```python
from build123d import *

# Parameters (mm, degrees)
SKETCH1_W            = 300
SKETCH1_H            = 20
BOSS_EXTRUDE1_DEPTH  = 8
SKETCH2_W            = 34
SKETCH2_H            = 8
BOSS_EXTRUDE2_DEPTH  = 9
SKETCH3_W            = 34
SKETCH3_H            = 8
BOSS_EXTRUDE3_DEPTH  = 9
SKETCH4_R            = 1.65
CUT_EXTRUDE1_DEPTH   = 302.504560496
SKETCH5_W            = 25
SKETCH5_H            = 8
BOSS_EXTRUDE4_DEPTH  = 17
SKETCH6_W            = 25
SKETCH6_H            = 8
BOSS_EXTRUDE5_DEPTH  = 17
SKETCH7_W            = 10
SKETCH7_H            = 38
CUT_EXTRUDE2_DEPTH   = 303.37890138
SKETCH8_W            = 7
SKETCH8_H            = 16
CUT_EXTRUDE3_DEPTH   = 4
CUT_EXTRUDE4_DEPTH   = 7
BOSS_EXTRUDE6_DEPTH  = 10
SKETCH12_W           = 8
SKETCH12_H           = 8
BOSS_EXTRUDE7_DEPTH  = 17
SKETCH13_R           = 1.7
CUT_EXTRUDE6_DEPTH   = 305.926220585
SKETCH14_W           = 20
SKETCH14_H           = 13
BOSS_EXTRUDE8_DEPTH  = 12
SKETCH15_R           = 1.6
CUT_EXTRUDE7_DEPTH   = 20
SKETCH16_W           = 20
SKETCH16_H           = 13
BOSS_EXTRUDE9_DEPTH  = 12
SKETCH17_R           = 1.6
CUT_EXTRUDE8_DEPTH   = 20
SKETCH18_W           = 20
SKETCH18_H           = 13
BOSS_EXTRUDE10_DEPTH = 12
SKETCH19_R           = 1.65
CUT_EXTRUDE9_DEPTH   = 20
SKETCH20_W           = 20
SKETCH20_H           = 13
BOSS_EXTRUDE11_DEPTH = 12
SKETCH21_R           = 1.65
CUT_EXTRUDE10_DEPTH  = 20
FILLET6_R            = 3
SKETCH22_W           = 123.750788161
SKETCH22_H           = 72.639217631
CUT_EXTRUDE11_DEPTH  = 244
SKETCH23_R           = 1.575
CUT_EXTRUDE12_DEPTH  = 71.611613776
FILLET7_R            = 3
SKETCH24_W           = 5.5
SKETCH24_H           = 78.243551934
CUT_EXTRUDE13_DEPTH  = 0.8
SKETCH25_W           = 20
SKETCH25_H           = 5.75655834
CUT_EXTRUDE14_DEPTH  = 0.5
SKETCH26_W           = 20
SKETCH26_H           = 21.459079842
CUT_EXTRUDE15_DEPTH  = 0.5


with BuildPart() as part:
    # Sketch1 → Boss-Extrude1 (new body)
    with BuildSketch(Plane(origin=(0, 0, 0), x_dir=(1, 0, 0), z_dir=(0, 1, 0))):
        with Locations((150, -10)):
            Rectangle(SKETCH1_W, SKETCH1_H)
    extrude(amount=BOSS_EXTRUDE1_DEPTH)

    # Sketch2 → Boss-Extrude2 (add)
    with BuildSketch(Plane.XY.offset(20)):
        with Locations((17, 4)):
            Rectangle(SKETCH2_W, SKETCH2_H)
        with Locations((283, 4)):
            Rectangle(SKETCH2_W, SKETCH2_H)
    extrude(amount=BOSS_EXTRUDE2_DEPTH)

    # Sketch3 → Boss-Extrude3 (add)
    with BuildSketch(Plane(origin=(0, 0, 0), x_dir=(-1, 0, 0), z_dir=(0, 0, -1))):
        with Locations((-17, 4)):
            Rectangle(SKETCH3_W, SKETCH3_H)
        with Locations((-283, 4)):
            Rectangle(SKETCH3_W, SKETCH3_H)
    extrude(amount=BOSS_EXTRUDE3_DEPTH)

    # Sketch4 → Cut-Extrude1 (cut, through all)
    with BuildSketch(Plane(origin=(0, 8, 0), x_dir=(1, 0, 0), z_dir=(0, 1, 0))):
        with Locations(Location((4, 5, 0), (0, 0, 270))):
            Circle(SKETCH4_R)
        with Locations(Location((30, 5, 0), (0, 0, 270))):
            Circle(SKETCH4_R)
        with Locations(Location((30, -25, 0), (0, 0, 270))):
            Circle(SKETCH4_R)
        with Locations(Location((4, -25, 0), (0, 0, 270))):
            Circle(SKETCH4_R)
        with Locations(Location((296, -25, 0), (0, 0, 270))):
            Circle(SKETCH4_R)
        with Locations(Location((296, 5, 0), (0, 0, 270))):
            Circle(SKETCH4_R)
        with Locations(Location((270, -25, 0), (0, 0, 270))):
            Circle(SKETCH4_R)
        with Locations(Location((270, 5, 0), (0, 0, 270))):
            Circle(SKETCH4_R)
    extrude(amount=-CUT_EXTRUDE1_DEPTH, mode=Mode.SUBTRACT)

    # Sketch5 → Boss-Extrude4 (add)
    with BuildSketch(Plane.XY.offset(20)):
        with Locations((253.5, 4)):
            Rectangle(SKETCH5_W, SKETCH5_H)
    extrude(amount=BOSS_EXTRUDE4_DEPTH)

    # Sketch6 → Boss-Extrude5 (add)
    with BuildSketch(Plane(origin=(0, 0, 0), x_dir=(-1, 0, 0), z_dir=(0, 0, -1))):
        with Locations((-253.5, 4)):
            Rectangle(SKETCH6_W, SKETCH6_H)
    extrude(amount=BOSS_EXTRUDE5_DEPTH)

    # Sketch7 → Cut-Extrude2 (cut, through all)
    with BuildSketch(Plane(origin=(0, 8, 0), x_dir=(1, 0, 0), z_dir=(0, 1, 0))):
        with Locations((254, -10)):
            Rectangle(SKETCH7_W, SKETCH7_H)
    extrude(amount=-CUT_EXTRUDE2_DEPTH, mode=Mode.SUBTRACT)

    # Sketch8 → Cut-Extrude3 (cut)
    with BuildSketch(Plane(origin=(0, 8, 0), x_dir=(1, 0, 0), z_dir=(0, 1, 0))):
        with Locations((262.5, -10)):
            Rectangle(SKETCH8_W, SKETCH8_H)
    extrude(amount=-CUT_EXTRUDE3_DEPTH, mode=Mode.SUBTRACT)

    # Sketch9 → Cut-Extrude4 (cut)
    with BuildSketch(Plane.ZY.offset(-259)):
        Polygon((18, 4), (22, 8), (18, 8), align=None)
        Polygon((2, 4), (-2, 8), (2, 8), align=None)
    extrude(amount=-CUT_EXTRUDE4_DEPTH, mode=Mode.SUBTRACT)

    # Sketch10 → Boss-Extrude6 (add)
    with BuildSketch(Plane.ZY.offset(-259)):
        Polygon((-2, 0), (-9, 8), (-9, 0), align=None)
        Polygon((29, 8), (22, 0), (29, 0), align=None)
    extrude(amount=BOSS_EXTRUDE6_DEPTH)

    # Sketch12 → Boss-Extrude7 (add)
    with BuildSketch(Plane.XY.offset(37)):
        with Locations((245, 4)):
            Rectangle(SKETCH12_W, SKETCH12_H)
    extrude(amount=BOSS_EXTRUDE7_DEPTH)

    # Sketch13 → Cut-Extrude6 (cut, through all)
    with BuildSketch(Plane(origin=(0, 8, 0), x_dir=(1, 0, 0), z_dir=(0, 1, 0))):
        with Locations(Location((245, -50, 0), (0, 0, 270))):
            Circle(SKETCH13_R)
        with Locations(Location((245, -18, 0), (0, 0, 270))):
            Circle(SKETCH13_R)
    extrude(amount=-CUT_EXTRUDE6_DEPTH, mode=Mode.SUBTRACT)

    # Sketch14 → Boss-Extrude8 (add)
    with BuildSketch(Plane.XY.offset(29)):
        with Locations((285, 6.5)):
            Rectangle(SKETCH14_W, SKETCH14_H)
    extrude(amount=BOSS_EXTRUDE8_DEPTH)

    # Sketch15 → Cut-Extrude7 (cut)
    with BuildSketch(Plane(origin=(295, 0, 0), x_dir=(0, 0, -1), z_dir=(1, 0, 0))):
        with Locations((-35, 8)):
            Circle(SKETCH15_R)
    extrude(amount=-CUT_EXTRUDE7_DEPTH, mode=Mode.SUBTRACT)

    # Sketch16 → Boss-Extrude9 (add)
    with BuildSketch(Plane(origin=(0, 0, -9), x_dir=(-1, 0, 0), z_dir=(0, 0, -1))):
        with Locations((-285, 6.5)):
            Rectangle(SKETCH16_W, SKETCH16_H)
    extrude(amount=BOSS_EXTRUDE9_DEPTH)

    # Sketch17 → Cut-Extrude8 (cut)
    with BuildSketch(Plane(origin=(295, 0, 0), x_dir=(0, 0, -1), z_dir=(1, 0, 0))):
        with Locations((15, 8)):
            Circle(SKETCH17_R)
    extrude(amount=-CUT_EXTRUDE8_DEPTH, mode=Mode.SUBTRACT)

    # Sketch18 → Boss-Extrude10 (add)
    with BuildSketch(Plane(origin=(0, 0, -9), x_dir=(-1, 0, 0), z_dir=(0, 0, -1))):
        with Locations((-15, 6.5)):
            Rectangle(SKETCH18_W, SKETCH18_H)
    extrude(amount=BOSS_EXTRUDE10_DEPTH)

    # Sketch19 → Cut-Extrude9 (cut)
    with BuildSketch(Plane.ZY.offset(-5)):
        with Locations((-15, 8)):
            Circle(SKETCH19_R)
    extrude(amount=-CUT_EXTRUDE9_DEPTH, mode=Mode.SUBTRACT)

    # Sketch20 → Boss-Extrude11 (add)
    with BuildSketch(Plane.XY.offset(29)):
        with Locations((15, 6.5)):
            Rectangle(SKETCH20_W, SKETCH20_H)
    extrude(amount=BOSS_EXTRUDE11_DEPTH)

    # Sketch21 → Cut-Extrude10 (cut)
    with BuildSketch(Plane.ZY.offset(-5)):
        with Locations((35, 8)):
            Circle(SKETCH21_R)
    extrude(amount=-CUT_EXTRUDE10_DEPTH, mode=Mode.SUBTRACT)

    # Fillet6
    fillet6_edges = [part.edges().sort_by_distance(p)[0] for p in [
        (285, 13, 29),
        (285, 13, 41),
        (285, 13, -9),
        (285, 13, -21),
        (15, 13, -9),
        (15, 13, -21),
        (15, 13, 29),
        (15, 13, 41),
    ]]
    fillet(fillet6_edges, radius=FILLET6_R)

    # Sketch22 → Cut-Extrude11 (cut)
    with BuildSketch(Plane(origin=(300, 0, 0), x_dir=(0, 0, -1), z_dir=(1, 0, 0))):
        with Locations((-10.128058827, -1.301866478)):
            Rectangle(SKETCH22_W, SKETCH22_H)
    extrude(amount=-CUT_EXTRUDE11_DEPTH, mode=Mode.SUBTRACT)

    # Sketch23 → Cut-Extrude12 (cut, through all)
    with BuildSketch(Plane(origin=(0, 0, 0), x_dir=(-1, 0, 0), z_dir=(0, -1, 0))):
        with Locations(Location((-51, -5, 0), (0, 0, 90))):
            Circle(SKETCH23_R)
        with Locations(Location((-51, -15, 0), (0, 0, 90))):
            Circle(SKETCH23_R)
        with Locations(Location((-43, -5, 0), (0, 0, 90))):
            Circle(SKETCH23_R)
        with Locations(Location((-43, -15, 0), (0, 0, 90))):
            Circle(SKETCH23_R)
    extrude(amount=-CUT_EXTRUDE12_DEPTH, mode=Mode.SUBTRACT)

    # Fillet7
    fillet7_edges = [part.edges().sort_by_distance(p)[0] for p in [
        (0, 4, 29),
        (34, 4, 29),
        (0, 4, -9),
        (34, 4, -9),
    ]]
    fillet(fillet7_edges, radius=FILLET7_R)

    # Sketch24 → Cut-Extrude13 (cut)
    with BuildSketch(Plane(origin=(0, 13, 0), x_dir=(1, 0, 0), z_dir=(0, 1, 0))):
        with Locations((15, -9.577024089)):
            Rectangle(SKETCH24_W, SKETCH24_H)
    extrude(amount=-CUT_EXTRUDE13_DEPTH, mode=Mode.SUBTRACT)

    # Sketch25 → Cut-Extrude14 (cut)
    with BuildSketch(Plane(origin=(0, 0, 29), x_dir=(-1, 0, 0), z_dir=(0, 0, -1))):
        with Locations((-15, 10.87827917)):
            Rectangle(SKETCH25_W, SKETCH25_H)
    extrude(amount=-CUT_EXTRUDE14_DEPTH, mode=Mode.SUBTRACT)

    # Sketch26 → Cut-Extrude15 (cut)
    with BuildSketch(Plane.XY.offset(-9)):
        with Locations((15, 18.729539921)):
            Rectangle(SKETCH26_W, SKETCH26_H)
    extrude(amount=-CUT_EXTRUDE15_DEPTH, mode=Mode.SUBTRACT)


solid = part.part
```
Here's how the part is built. I have some questions about the finished solid (model axes, mm). A direction names the side the tool comes from. Give positions to 0.01 mm unless a question says otherwise; leave off trailing zeros. Order: outer loops, then holes, each group sorted by start corner. A loop starts at its lowest first (then second) coordinate and runs counter-clockwise, first axis right, second up. Notation, with made-up numbers: (27.5, 5) - (46.5, 5) arc R19 ccw to (46.5, 22) - close; hole circle Ø5 at (-27.5, 15.25). An arc over 180 degrees is marked (long way). Answer as a JSON object with one key per item and string values. Group by question number.
Item 1: If we section it at A-A on x = 43: Please give me the cut outline in (y, z) (3 decimals), and give its area (3 significant figures).
Item 2: If we section it at D-D on z = 15: Please give me the cut outline in (x, y) (3 decimals).
Item 3: Which directions (+Z, -Z, +X, -X, +Y, -Y) give clear straight access to the entire face, cutting with the end or side of a thin tool? Please do faces 4 (the flat face through (15, 10, -9.5)), 5 (the flat face through (28, 4, 29)), 6 (the flat face through (4, 4, -9)), 7 (the flat face through (5, 5, 35)).
Item 4: For P1, Ø5, axis at x = 30.5, z = 0.5, coming from the +Y side; P2, Ø6.5, axis at x = 50, y = 5, coming from the -Z side; P3, Ø3, axis at x = 4, z = -5, coming from the -Y side; P4, Ø4.5, axis at y = 8, z = 35, coming from the -X side, each with a flat end and sliding along its axis, tell me the tip position at first contact or that it passes through.
Item 5: If we mould it in two halves opening along X, with no side actions, what happens to faces 1 (the flat face through (15, 12.2, 35)), 2 (the cylindrical face through (14.86, 11.69, -20.48)), 3 (the cylindrical face through (0.9, 4.06, 28.14))? For each: pulls with the +X half, pulls with the -X half, needs draft (parallel to the pull), parting line crosses it, or undercut.
Item 6: Please list where these lines run through material, in increasing order: probe 1 along X at (y, z) = (5.75, 5) (3 decimals); probe 2 along Z at (x, y) = (3, 2.25); probe 3 along Z at (x, y) = (5.5, 1).
Item 7: If we section it at B-B on z = -15: Please give me the cut outline in (x, y).
Item 8: If we section it at C-C on y = 3.5: Give the number of separate pieces and of enclosed holes in the cut face, and give its area (3 significant figures).
Result set:
{
 "1": {"outline": "(0, 0) - (8, 0) - (8, 3.425) - (0, 3.425) - close; (0, 6.575) - (8, 6.575) - (8, 13.425) - (0, 13.425) - close; (0, 16.575) - (8, 16.575) - (8, 20) - (0, 20) - close", "area": "110 mm²"},
 "2": {"outline": "(0, 0) - (41.425, 0) - (41.425, 8) - (0, 8) - close; (44.575, 0) - (49.425, 0) - (49.425, 8) - (44.575, 8) - close; (52.575, 0) - (56, 0) - (56, 8) - (52.575, 8) - close"},
 "3": {"face 4": "+X, -X, +Y", "face 5": "+Z, +X, +Y, -Y", "face 6": "-Z, -X, +Y, -Y", "face 7": "+Z, -X, +Y, -Y"},
 "4": {"P1": "y = 8", "P2": "z = 0", "P3": "through", "P4": "x = 5"},
 "5": {"face 1": "undercut", "face 2": "needs draft", "face 3": "pulls with the -X half"},
 "6": {"probe 1": "0 to 41.425, 44.575 to 49.425, 52.575 to 56", "probe 2": "-9 to -6.31, -3.69 to 23.69, 26.31 to 29", "probe 3": "-21 to -5.69, -4.31 to 24.31, 25.69 to 41"},
 "7": {"outline": "(5, 0) - (25, 0) - (25, 6.35) - (5, 6.35) - close; (5, 9.65) - (25, 9.65) - (25, 13) - (17.75, 13) - (17.75, 12.2) - (12.25, 12.2) - (12.25, 13) - (5, 13) - close"},
 "8": {"separate pieces": "1", "enclosed holes": "8", "area": "2,140 mm²"}
}
